```python
from build123d import *

# Parameters (mm, degrees)
SKETCH_5_W         = 1.75
SKETCH_5_H         = 47
SKETCH_6_W         = 1.75
SKETCH_6_H         = 47
SKETCH_7_W         = 9
SKETCH_7_H         = 1.75
LEFT_ORNER_ANGLE   = 90
RIGHT_CORNER_ANGLE = 90
SKETCH_11_R        = 0.5
SKETCH_13_R        = 0.5


with BuildPart() as part:
    # 草圖5 → left (revolve)
    with BuildSketch(Plane(origin=(0, 0, 0), x_dir=(1, 0, 0), z_dir=(0, 1, 0))):
        with Locations((-3.625, -23.5)):
            Rectangle(SKETCH_5_W, SKETCH_5_H)
    revolve(axis=Axis((-4.5, 0, 47), (0, 0, -1)))



with BuildPart() as body_2:
    # 草圖6 → right (revolve)
    with BuildSketch(Plane(origin=(0, 0, 0), x_dir=(1, 0, 0), z_dir=(0, 1, 0))):
        with Locations((5.375, -23.5)):
            Rectangle(SKETCH_6_W, SKETCH_6_H)
    revolve(axis=Axis((4.5, 0, 0), (0, 0, 1)))


with BuildPart() as part_1:
    add(part.part)

    add(body_2.part)  # down merges body 2
    # 草圖7 → down (revolve)
    with BuildSketch(Plane(origin=(0, 0, 0), x_dir=(1, 0, 0), z_dir=(0, 1, 0))):
        with Locations((0, 0.875)):
            Rectangle(SKETCH_7_W, SKETCH_7_H)
    revolve(axis=Axis((-4.5, 0, 0), (1, 0, 0)))

    # 草圖8 → left_orner (revolve)
    with BuildSketch(Plane(origin=(0, 0, 0), x_dir=(-1, 0, 0), z_dir=(0, 0, -1))):
        with BuildLine():
            Line((4.5, -1.75), (4.5, 1.75))
            ThreePointArc((4.5, 1.75), (6.25, 0), (4.5, -1.75))
        make_face()
    revolve(axis=Axis((-4.5, -1.75, 0), (0, -1, 0)), revolution_arc=LEFT_ORNER_ANGLE)

    # 草圖9 → right_corner (revolve)
    with BuildSketch(Plane(origin=(0, 0, 0), x_dir=(-1, 0, 0), z_dir=(0, 0, -1))):
        with BuildLine():
            Line((-4.5, -1.75), (-4.5, 1.75))
            ThreePointArc((-4.5, 1.75), (-6.25, 0), (-4.5, -1.75))
        make_face()
    revolve(axis=Axis((4.5, -1.75, 0), (0, 1, 0)), revolution_arc=RIGHT_CORNER_ANGLE)

    # 草圖10 → up (revolve)
    with BuildSketch(Plane(origin=(0, 0, 0), x_dir=(1, 0, 0), z_dir=(0, 1, 0))):
        Polygon((-4.131218222, -29.718048494), (-4.131218222, -31.459518002), (4.131218222, -29.623421015), (4.131218222, -27.881951506), align=None)
    revolve(axis=Axis((-4.5, 0, 29.8), (0.97618706, 0, -0.216930458)))

    # inside: sweep along a path in 草圖12
    with BuildLine(Plane(origin=(0, 0, 0), x_dir=(1, 0, 0), z_dir=(0, 1, 0))) as inside_path:
        Line((-4.5, -47), (-4.5, -1))
        ThreePointArc((-4.5, -1), (-4.207106781, -0.292893219), (-3.5, 0))
        Line((-3.5, 0), (3.5, 0))
        ThreePointArc((3.5, 0), (4.207106781, -0.292893219), (4.5, -1))
        Line((4.5, -1), (4.5, -47))
    # 草圖11 → inside (sweep, cut)
    with BuildSketch(Plane.XY.offset(47)):
        with Locations((-4.5, 0)):
            Circle(SKETCH_11_R)
    sweep(path=inside_path.line, mode=Mode.SUBTRACT)

    # up_inside: sweep along a path in 草圖14
    with BuildLine(Plane(origin=(0, 0, 0), x_dir=(1, 0, 0), z_dir=(0, 1, 0))) as up_inside_path:
        Line((4.5, -27.8), (-4.5, -29.8))
    # 草圖13 → up_inside (sweep, cut)
    with BuildSketch(Plane(origin=(4.5, 0, 0), x_dir=(0, 0, -1), z_dir=(1, 0, 0))):
        with Locations((-27.8, 0)):
            Circle(SKETCH_13_R)
    sweep(path=up_inside_path.line, mode=Mode.SUBTRACT)


solid = part_1.part
```
Can you work these out from the model? Positions are in its coordinate system, mm. A direction names the side the tool comes from. Coordinates: 2 decimals unless noted, no trailing zeros. Write each loop counter-clockwise with the first axis right and the second up, starting at its lowest first coordinate (ties: lowest second). Pieces come first, ordered by that corner, then holes. Notation, with made-up numbers: M 14.5,78.5 L 42.5,78.5 A8 ccw 42.5,84.5 Z; hole C 63,64 d6. An arc over 180 degrees is marked long. Write item = value, one per line. Start each with the question number.
Q1. Thinking about a two-plate mould opening in X: for faces 4 (the face through (-6.25, -0.08, 23.17)), 5 (the face through (3.7, 0, 47)), which applies, released by +X, released by -X, zero draft, split by the parting line, or undercut?
Q2. If we section it at A-A, the plane z = 38.5: Write out the boundary of the cut face in (x, y).
Q3. On a 3-axis mill with a long thin cutter (end or side, diameter ignored), from which of +Z, -Z, +X, -X, +Y, -Y can I reach the whole of each face in a straight line? I mean faces 1 (the face through (-5.3, 0, 47)), 2 (the face through (6.169, 0.526, 23.171)), 3 (the face through (5, 0, 24)). Say none if no direction works.
Q4. I'm going to push flat-ended pins straight in: pin 1 (2 mm diameter, centred on x = 0, y = -1.5, fed in from +Z); pin 2 (1.5 mm diameter, centred on y = -1, z = 35.5, fed in from -X). Where does each tip first touch, or does it pass through?
Q5. If we section it at B-B, the plane y = 0: State how many separate pieces and enclosed holes the cut face has, then the cut area to 3 significant figures.
Q6. If I drill on L1, parallel to X at y = 0, z = 14; L2, parallel to Z at x = -3, y = 0.15; L3, parallel to Z at x = 0.75, y = -0.35, over which ranges is the centre line in solid material (lowest first)? Write a range as [from, to].
Q7. If we section it at D-D, the plane x = 5.5: Write out the boundary of the cut face in (y, z), then the cut area to 3 significant figures.
Check sheet entries:
q1.face_4 = undercut
q1.face_5 = zero draft
q2.outline = C -4.5,0 d3.5; C 4.5,0 d3.5; hole C -4.5,0 d1; hole C 4.5,0 d1
q3.face_1 = +Z, +X, -X, +Y, -Y
q3.face_2 = none
q3.face_3 = +Z
q4.pin_1 = 30.53
q4.pin_2 = -6.23
q5.separate_pieces = 3
q5.enclosed_holes = 1
q5.area = 268 mm²
q6.L1 = [-6.25, -5], [-4, -2.75], [2.75, 4], [5, 6.25]
q6.L2 = [-1.74, -0.48], [0.48, 28.99], [29.94, 47]
q6.L3 = [-1.71, -0.36], [0.36, 1.71], [26.93, 28.28], [28.99, 30.34]
q7.outline = M -1.44,0 A1.44 ccw 1.44,0 L 1.44,47 L -1.44,47 Z
q7.area = 138 mm²
